Input: dimensioned drawing with shaded views. Units: mm. Origin: part minimum x, y, z. A direction names the side the tool comes from. Give positions to 0.01 mm unless a question says otherwise; leave off trailing zeros. Order: outer loops, then holes, each group sorted by start corner. A loop starts at its lowest first (then second) coordinate and runs counter-clockwise, first axis right, second up. Notation, with made-up numbers: (-10.5, 9) -> (30.5, 9) arc R7 ccw to (30.5, 17) -> close; hole circle Ø1 at (-33, 7.5). An arc over 180 degrees is marked (long way). One line per question, with ' | ' between items. Start each with the question number.
(1) First-contact query: pin 1 Ø1.6 at (x, z) = (11.5, 16.5) entering from -Y; pin 2 Ø6 at (x, z) = (5.5, 17.5) entering from +Y; pin 3 Ø12 at (y, z) = (33, 6.5) entering from -X. Flat tips, straight axial feed; report the tip coordinate or a pass-through.
(2) Section D-D (x = 4). Return loops of the section in (y, z), then the cut area to 3 significant figures.
(3) Section B-B (x = 20). Return loops of the section in (y, z).
(4) Section C-C (z = 16). Return loops of the section in (x, y), then the cut area to 3 significant figures.
(5) Set-up query: the marked faces 1 and 2. Return all of +Z, -Z, +X, -X, +Y, -Y with unobstructed straight access to the full face (end or side cutting, diameter ignored); none if empty.
(6) Ray query, L1, parallel to X at y = 6, z = 16; L2, parallel to Z at x = 21, y = 10.5; L3, parallel to X at y = 36.5, z = 1.75. Return the intervals inside material, ascending.
(7) Section A-A (y = 4). Return loops of the section in (x, z), then the cut area to 3 significant figures.
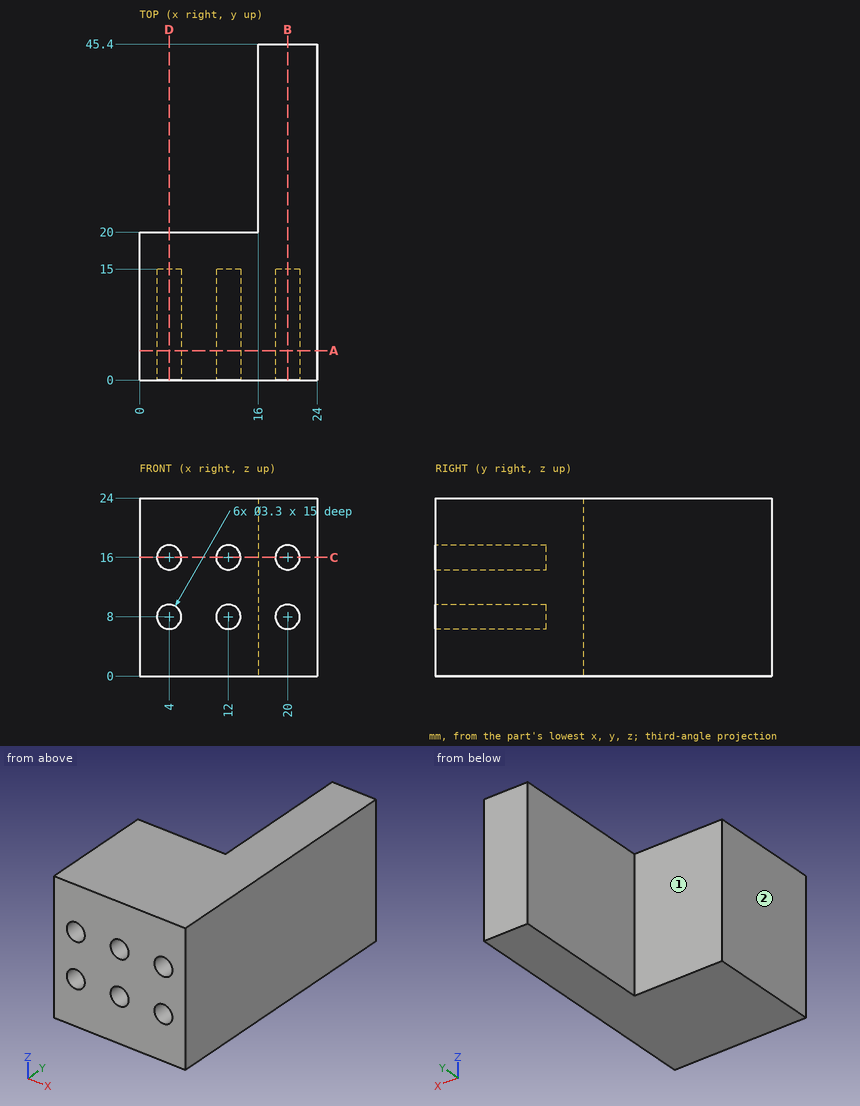
Response:
1) pin 1: stops at y = 15 | pin 2: stops at y = 20 | pin 3: stops at x = 16
2) outline: (0, 0) -> (20, 0) -> (20, 24) -> (0, 24) -> (0, 17.65) -> (15, 17.65) -> (15, 14.35) -> (0, 14.35) -> (0, 9.65) -> (15, 9.65) -> (15, 6.35) -> (0, 6.35) -> close | area: 381 mm^2
3) outline: (0, 0) -> (45.4, 0) -> (45.4, 24) -> (0, 24) -> (0, 17.65) -> (15, 17.65) -> (15, 14.35) -> (0, 14.35) -> (0, 9.65) -> (15, 9.65) -> (15, 6.35) -> (0, 6.35) -> close
4) outline: (0, 0) -> (2.35, 0) -> (2.35, 15) -> (5.65, 15) -> (5.65, 0) -> (10.35, 0) -> (10.35, 15) -> (13.65, 15) -> (13.65, 0) -> (18.35, 0) -> (18.35, 15) -> (21.65, 15) -> (21.65, 0) -> (24, 0) -> (24, 45.4) -> (16, 45.4) -> (16, 20) -> (0, 20) -> close | area: 535 mm^2
5) face 1: +Z, -Z, -X, +Y | face 2: +Z, -Z, -X, +Y, -Y
6) L1: x = 0 to 2.35, 5.65 to 10.35, 13.65 to 18.35, 21.65 to 24 | L2: z = 0 to 6.69, 9.31 to 14.69, 17.31 to 24 | L3: x = 16 to 24
7) outline: (0, 0) -> (24, 0) -> (24, 24) -> (0, 24) -> close; hole circle Ø3.3 at (4, 8); hole circle Ø3.3 at (4, 16); hole circle Ø3.3 at (12, 8); hole circle Ø3.3 at (12, 16); hole circle Ø3.3 at (20, 8); hole circle Ø3.3 at (20, 16) | area: 525 mm^2
